The model under review builds one solid part; all positions refer to its coordinate system, in mm. A direction names the side the tool comes from. Coordinates: 2 decimals unless noted, no trailing zeros. Write each loop counter-clockwise with the first axis right and the second up, starting at its lowest first coordinate (ties: lowest second). Pieces come first, ordered by that corner, then holes. Notation, with made-up numbers: (-3.5, -6) -> (21.5, -6) arc R19 ccw to (21.5, 3) -> close; hole circle Ø11 at (37.5, 74). An arc over 180 degrees is marked (long way). Put each result on its own line as item: value. Start each with the question number.
from build123d import *

# Parameters (mm, degrees)
F0_R     = 2
F1_DEPTH = 100
F2_R     = 1.5
F3_DEPTH = 10


with BuildPart() as f1:
    # F0 (on Front) → F1 (new body)
    with BuildSketch(Plane.XZ):
        with BuildLine():
            ThreePointArc((15, 13.5), (14.56066, 14.56066), (13.5, 15))
            Line((13.5, 15), (4, 15))
            ThreePointArc((4, 15), (3.292893, 14.707107), (3, 14))
            Line((3, 14), (3, 13))
            ThreePointArc((3, 13), (3.292893, 12.292893), (4, 12))
            Line((4, 12), (7.464466, 12))
            ThreePointArc((7.464466, 12), (8.388346, 11.382683), (8.171573, 10.292893))
            Line((8.171573, 10.292893), (3.318019, 5.43934))
            ThreePointArc((3.318019, 5.43934), (2.831384, 5.114181), (2.257359, 5))
            Line((2.257359, 5), (-2.257359, 5))
            ThreePointArc((-2.257359, 5), (-2.831384, 5.114181), (-3.318019, 5.43934))
            Line((-3.318019, 5.43934), (-8.171573, 10.292893))
            ThreePointArc((-8.171573, 10.292893), (-8.388346, 11.382683), (-7.464466, 12))
            Line((-7.464466, 12), (-4, 12))
            ThreePointArc((-4, 12), (-3.292893, 12.292893), (-3, 13))
            Line((-3, 13), (-3, 14))
            ThreePointArc((-3, 14), (-3.292893, 14.707107), (-4, 15))
            Line((-4, 15), (-13.5, 15))
            ThreePointArc((-13.5, 15), (-14.56066, 14.56066), (-15, 13.5))
            Line((-15, 13.5), (-15, 4))
            ThreePointArc((-15, 4), (-14.707107, 3.292893), (-14, 3))
            Line((-14, 3), (-13, 3))
            ThreePointArc((-13, 3), (-12.292893, 3.292893), (-12, 4))
            Line((-12, 4), (-12, 7.464466))
            ThreePointArc((-12, 7.464466), (-11.382683, 8.388346), (-10.292893, 8.171573))
            Line((-10.292893, 8.171573), (-5.43934, 3.318019))
            ThreePointArc((-5.43934, 3.318019), (-5.114181, 2.831384), (-5, 2.257359))
            Line((-5, 2.257359), (-5, -2.257359))
            ThreePointArc((-5, -2.257359), (-5.114181, -2.831384), (-5.43934, -3.318019))
            Line((-5.43934, -3.318019), (-10.292893, -8.171573))
            ThreePointArc((-10.292893, -8.171573), (-11.382683, -8.388346), (-12, -7.464466))
            Line((-12, -7.464466), (-12, -4))
            ThreePointArc((-12, -4), (-12.292893, -3.292893), (-13, -3))
            Line((-13, -3), (-14, -3))
            ThreePointArc((-14, -3), (-14.707107, -3.292893), (-15, -4))
            Line((-15, -4), (-15, -13.5))
            ThreePointArc((-15, -13.5), (-14.56066, -14.56066), (-13.5, -15))
            Line((-13.5, -15), (-4, -15))
            ThreePointArc((-4, -15), (-3.292893, -14.707107), (-3, -14))
            Line((-3, -14), (-3, -13))
            ThreePointArc((-3, -13), (-3.292893, -12.292893), (-4, -12))
            Line((-4, -12), (-7.464466, -12))
            ThreePointArc((-7.464466, -12), (-8.388346, -11.382683), (-8.171573, -10.292893))
            Line((-8.171573, -10.292893), (-3.318019, -5.43934))
            ThreePointArc((-3.318019, -5.43934), (-2.831384, -5.114181), (-2.257359, -5))
            Line((-2.257359, -5), (2.257359, -5))
            ThreePointArc((2.257359, -5), (2.831384, -5.114181), (3.318019, -5.43934))
            Line((3.318019, -5.43934), (8.171573, -10.292893))
            ThreePointArc((8.171573, -10.292893), (8.388346, -11.382683), (7.464466, -12))
            Line((7.464466, -12), (4, -12))
            ThreePointArc((4, -12), (3.292893, -12.292893), (3, -13))
            Line((3, -13), (3, -14))
            ThreePointArc((3, -14), (3.292893, -14.707107), (4, -15))
            Line((4, -15), (13.5, -15))
            ThreePointArc((13.5, -15), (14.56066, -14.56066), (15, -13.5))
            Line((15, -13.5), (15, -4))
            ThreePointArc((15, -4), (14.707107, -3.292893), (14, -3))
            Line((14, -3), (13, -3))
            ThreePointArc((13, -3), (12.292893, -3.292893), (12, -4))
            Line((12, -4), (12, -7.464466))
            ThreePointArc((12, -7.464466), (11.382683, -8.388346), (10.292893, -8.171573))
            Line((10.292893, -8.171573), (5.43934, -3.318019))
            ThreePointArc((5.43934, -3.318019), (5.114181, -2.831384), (5, -2.257359))
            Line((5, -2.257359), (5, 2.257359))
            ThreePointArc((5, 2.257359), (5.114181, 2.831384), (5.43934, 3.318019))
            Line((5.43934, 3.318019), (10.292893, 8.171573))
            ThreePointArc((10.292893, 8.171573), (11.382683, 8.388346), (12, 7.464466))
            Line((12, 7.464466), (12, 4))
            ThreePointArc((12, 4), (12.292893, 3.292893), (13, 3))
            Line((13, 3), (14, 3))
            ThreePointArc((14, 3), (14.707107, 3.292893), (15, 4))
            Line((15, 4), (15, 13.5))
        make_face()
        Circle(F0_R, mode=Mode.SUBTRACT)
    extrude(amount=-F1_DEPTH)

    # F2 (on face) → F3 (cut)
    with BuildSketch(Plane.XY.offset(5)):
        with Locations((0, 50)):
            Circle(F2_R)
    extrude(amount=-F3_DEPTH, mode=Mode.SUBTRACT)


solid = f1.part
1. Tool access review of faces 1 (the flat face through (1.5, 49.3, -5)), 2 (the flat face through (-15, 49, 9)), 3 (the flat face through (5, 49, 0)), 4 (the cylindrical face through (-11.4, 49.3, 8.38)): name each direction out of +Z, -Z, +X, -X, +Y, -Y from which nothing blocks a thin tool from reaching the whole face with its end or side.
2. Wall thickness on line 1 (Z direction, x = 13, y = 50.5); line 2 (X direction, y = 50, z = -3.2); line 3 (Z direction, x = 3.5, y = 70): over which ranges is each line inside the solid? List them lowest first. Write a range as from..to.
3. Insertion check: P1, Ø5, axis at x = 0, y = 50, coming from the +Z side; P2, Ø1.4, axis at y = 62, z = 0.5, coming from the -X side; P3, Ø3.5, axis at x = -0.5, y = 64, coming from the -Z side. Each pin has a flat end and moves straight along its axis. Give the tip position at first contact, or say it passes through.
4. Consider section A-A on x = 0. State the section outline as (y, z) points, then the cut area to 3 significant figures.
5. The part is to be moulded in two halves that separate along X. For faces 5 (the cylindrical face through (11.4, 49.3, -8.38)), 6 (the flat face through (-15, 49, -9)), 7 (the flat face through (-4, 0, 0)), say which applies: released by +X, released by -X, zero draft, split by the parting line, or undercut.
6. Consider section B-B on z = 0. State the section outline as (x, y) points.
Output values:
1. face 1: -Z, +Y, -Y
1. face 2: +Z, -Z, -X, +Y, -Y
1. face 3: +X, +Y, -Y
1. face 4: +Y, -Y
2. line 1: z = -15..-3, 3..15
2. line 2: x = -14.6..-12.4, -5.33..-1.5, 1.5..5.33, 12.4..14.6
2. line 3: z = -14.87..-12.13, -5.62..5.62, 12.13..14.87
3. P1: stops at z = 5.02
3. P2: stops at x = -5
3. P3: stops at z = -5
4. outline: (0, -5) -> (48.5, -5) -> (48.5, -2) -> (0, -2) -> close; (0, 2) -> (48.5, 2) -> (48.5, 5) -> (0, 5) -> close; (51.5, -5) -> (100, -5) -> (100, -2) -> (51.5, -2) -> close; (51.5, 2) -> (100, 2) -> (100, 5) -> (51.5, 5) -> close
4. area: 582 mm^2
5. face 5: undercut
5. face 6: released by -X
5. face 7: zero draft
6. outline: (-5, 0) -> (-2, 0) -> (-2, 100) -> (-5, 100) -> close; (2, 0) -> (5, 0) -> (5, 100) -> (2, 100) -> close
